Check sheet for the modelled part. Datum: model origin and axes. Units: mm. A direction names the side the tool comes from. Give positions to 0.01 mm unless a question says otherwise; leave off trailing zeros. Order: outer loops, then holes, each group sorted by start corner. A loop starts at its lowest first (then second) coordinate and runs counter-clockwise, first axis right, second up.
from build123d import *

# Parameters (mm, degrees)
SKETCH_W        = 100
SKETCH_H        = 55
PAD_DEPTH       = 6
SKETCH001_W     = 90.2
SKETCH001_H     = 50.2
POCKET_DEPTH    = 3
SKETCH002_R     = 2
PAD001_DEPTH    = 3
SKETCH003_R     = 0.9
PAD002_DEPTH    = 1
SKETCH004_W     = 3
SKETCH004_H     = 1.5
SKETCH004_H_2   = 3
POCKET001_DEPTH = 6
SKETCH005_W     = 3
SKETCH005_H     = 5
SKETCH005_H_2   = 21
POCKET002_DEPTH = 3
SKETCH006_W     = 5
SKETCH006_H     = 2
POCKET003_DEPTH = 1
SKETCH007_W     = 5
SKETCH007_H     = 2
POCKET004_DEPTH = 1
SKETCH008_R     = 16.5
POCKET005_DEPTH = 1
SKETCH009_R     = 2.25
SKETCH009_R_2   = 1.6
POCKET006_DEPTH = 2
SKETCH010_W     = 3
SKETCH010_H     = 5
PAD003_DEPTH    = 1
CHAMFER_SIZE    = 1


with BuildPart() as part:
    # Sketch → Pad (new body)
    with BuildSketch(Plane.XY):
        with Locations((-7, 0)):
            Rectangle(SKETCH_W, SKETCH_H)
    extrude(amount=PAD_DEPTH)

    # Sketch001 (on Face6 of Pad) → Pocket (cut)
    with BuildSketch(Plane.XY.offset(6)):
        with Locations((-10, 0)):
            Rectangle(SKETCH001_W, SKETCH001_H)
    extrude(amount=-POCKET_DEPTH, mode=Mode.SUBTRACT)

    # Sketch002 (on Face11 of Pocket) → Pad001 (join)
    with BuildSketch(Plane.XY.offset(3)):
        with Locations((-32.5, 22.5)):
            Circle(SKETCH002_R)
        with Locations((32.5, 22.5)):
            Circle(SKETCH002_R)
        with Locations((-32.5, -22.5)):
            Circle(SKETCH002_R)
        with Locations((32.5, -22.5)):
            Circle(SKETCH002_R)
    extrude(amount=PAD001_DEPTH)

    # Sketch003 (on Face19 of Pad001) → Pad002 (join)
    with BuildSketch(Plane.XY.offset(6)):
        with Locations((-32.5, 22.5)):
            Circle(SKETCH003_R)
        with Locations((32.5, 22.5)):
            Circle(SKETCH003_R)
        with Locations((-32.5, -22.5)):
            Circle(SKETCH003_R)
        with Locations((32.5, -22.5)):
            Circle(SKETCH003_R)
    extrude(amount=PAD002_DEPTH)

    # Sketch004 (on Face5 of Pad002) → Pocket001 (cut)
    with BuildSketch(Plane.XY.offset(6)):
        with Locations((39, 16.75)):
            Rectangle(SKETCH004_W, SKETCH004_H)
        with Locations((39, 9.5)):
            Rectangle(SKETCH004_W, SKETCH004_H_2)
        with Locations((39, 1.5)):
            Rectangle(SKETCH004_W, SKETCH004_H_2)
        with Locations((39, -5.75)):
            Rectangle(SKETCH004_W, SKETCH004_H)
        with Locations((39, -14.75)):
            Rectangle(SKETCH004_W, SKETCH004_H)
        with Locations((39, -21.25)):
            Rectangle(SKETCH004_W, SKETCH004_H)
    extrude(amount=-POCKET001_DEPTH, mode=Mode.SUBTRACT)

    # Sketch005 (on Face4 of Pocket001) → Pocket002 (cut)
    with BuildSketch(Plane(origin=(0, 0, 0), x_dir=(1, 0, 0), z_dir=(0, 0, -1))):
        with Locations((39, 18)):
            Rectangle(SKETCH005_W, SKETCH005_H)
        with Locations((39, -5.5)):
            Rectangle(SKETCH005_W, SKETCH005_H_2)
    extrude(amount=-POCKET002_DEPTH, mode=Mode.SUBTRACT)

    # Sketch006 (on Face6 of Pocket002) → Pocket003 (cut)
    with BuildSketch(Plane.XZ.offset(27.5)):
        with Locations((-18.5, 3)):
            Rectangle(SKETCH006_W, SKETCH006_H)
        with Locations((18.5, 3)):
            Rectangle(SKETCH006_W, SKETCH006_H)
    extrude(amount=-POCKET003_DEPTH, mode=Mode.SUBTRACT)

    # Sketch007 (on Face1 of Pocket003) → Pocket004 (cut)
    with BuildSketch(Plane(origin=(0, 27.5, 0), x_dir=(-1, 0, 0), z_dir=(0, 1, 0))):
        with Locations((-18.5, 3)):
            Rectangle(SKETCH007_W, SKETCH007_H)
        with Locations((18.5, 3)):
            Rectangle(SKETCH007_W, SKETCH007_H)
    extrude(amount=-POCKET004_DEPTH, mode=Mode.SUBTRACT)

    # Sketch008 (on Face3 of Pocket004) → Pocket005 (cut)
    with BuildSketch(Plane(origin=(0, 0, 0), x_dir=(1, 0, 0), z_dir=(0, 0, -1))):
        with Locations((-40, 0)):
            Circle(SKETCH008_R)
    extrude(amount=-POCKET005_DEPTH, mode=Mode.SUBTRACT)

    # Sketch009 (on Face70 of Pocket005) → Pocket006 (cut)
    with BuildSketch(Plane(origin=(0, 0, 1), x_dir=(1, 0, 0), z_dir=(0, 0, -1))):
        with Locations((-40, 6)):
            Circle(SKETCH009_R)
        with Locations((-40, -6)):
            Circle(SKETCH009_R)
        with Locations((-45, 0)):
            Circle(SKETCH009_R_2)
        with Locations((-35, 0)):
            Circle(SKETCH009_R_2)
    extrude(amount=-POCKET006_DEPTH, mode=Mode.SUBTRACT)

    # Sketch010 (on Face4 of Pocket006) → Pad003 (join)
    with BuildSketch(Plane.XY.offset(6)):
        with Locations((39, 13.5)):
            Rectangle(SKETCH010_W, SKETCH010_H)
        with Locations((39, -2.5)):
            Rectangle(SKETCH010_W, SKETCH010_H)
        with Locations((39, 5.5)):
            Rectangle(SKETCH010_W, SKETCH010_H)
        with Locations((39, -18)):
            Rectangle(SKETCH010_W, SKETCH010_H)
    extrude(amount=PAD003_DEPTH)

    # Chamfer
    chamfer_edges = [part.edges().sort_by_distance(p)[0] for p in [
        (-36.6, 0, 3),
        (-46.6, 0, 3),
    ]]
    chamfer(chamfer_edges, length=CHAMFER_SIZE)


solid = part.part
1) Section check D-D, the plane x = -25. Record the cut outline in (y, z), then the cut area to 3 significant figures.
Recorded:
outline: (-27.5, 0) - (-6.87, 0) - (-6.87, 1) - (6.87, 1) - (6.87, 0) - (27.5, 0) - (27.5, 6) - (25.1, 6) - (25.1, 3) - (-25.1, 3) - (-25.1, 6) - (-27.5, 6) - close
area: 166 mm2
2) Depth check by flat-ended pin: pin 1 Ø10 at (x, y) = (-7.5, 12.5) entering from +Z; pin 2 Ø2 at (x, y) = (-34, -10.5) entering from -Z. Enter the tip coordinate at first touch or a pass-through.
Recorded:
pin 1: stops at z = 3
pin 2: stops at z = 1
3) Section check C-C, the plane x = 22.5. Record the cut outline in (y, z), then the cut area to 3 significant figures.
Recorded:
outline: (-27.5, 0) - (27.5, 0) - (27.5, 6) - (25.1, 6) - (25.1, 3) - (-25.1, 3) - (-25.1, 6) - (-27.5, 6) - close
area: 179 mm2
4) Material ranges on L1, parallel to X at y = 0, z = 1.8; L2, parallel to X at y = 0, z = 0.65; L3, parallel to X at y = -9, z = 4.75, recorded low to high.
Recorded:
L1: x = -57 to -46.6, -43.4 to -36.6, -33.4 to 37.5, 40.5 to 43
L2: x = -57 to -56.5, -23.5 to 37.5, 40.5 to 43
L3: x = -57 to -55.1, 35.1 to 43
5) Section check B-B, the plane y = 6. Record the cut outline in (x, z).
Recorded:
outline: (-57, 0) - (-55.37, 0) - (-55.37, 1) - (-42.25, 1) - (-42.25, 3) - (-55.1, 3) - (-55.1, 6) - (-57, 6) - close; (-37.75, 1) - (-24.63, 1) - (-24.63, 0) - (37.5, 0) - (37.5, 3) - (40.5, 3) - (40.5, 0) - (43, 0) - (43, 6) - (40.5, 6) - (40.5, 7) - (37.5, 7) - (37.5, 6) - (35.1, 6) - (35.1, 3) - (-37.75, 3) - close
6) Draft check along Z on faces 5 (the face through (39, 6, 7)), 6 (the face through (39, -18, 3)), 7 (the face through (-19, -26.5, 3)), 8 (the face through (18, -26.5, 3)). Enter one of: +Z half, -Z half, draft (parallel to the pull), parting line (faces both ways), or undercut.
Recorded:
face 5: +Z half
face 6: -Z half
face 7: undercut
face 8: undercut
7) Section check A-A, the plane x = -40. Record the cut outline in (y, z), then the cut area to 3 significant figures.
Recorded:
outline: (-27.5, 0) - (-16.5, 0) - (-16.5, 1) - (-8.25, 1) - (-8.25, 3) - (-25.1, 3) - (-25.1, 6) - (-27.5, 6) - close; (-3.75, 1) - (3.75, 1) - (3.75, 3) - (-3.75, 3) - close; (8.25, 1) - (16.5, 1) - (16.5, 0) - (27.5, 0) - (27.5, 6) - (25.1, 6) - (25.1, 3) - (8.25, 3) - close
area: 128 mm2
8) Set-up check for faces 1 (the face through (32.38, 23.39, 6.49)), 2 (the face through (39, -18, 7)), 3 (the face through (37.5, 5, 2)), 4 (the face through (39, -6.5, 3)): record each of +Z, -Z, +X, -X, +Y, -Y from which the full face is reachable in a straight line by a thin tool's end or side.
Recorded:
face 1: +Z
face 2: +Z, +X, -X, +Y, -Y
face 3: -Z
face 4: +Z, -Z
